Part model, mm, in its own coordinate system. Face numbers are marked on the shaded views. A direction names the side the tool comes from. Give positions to 0.01 mm unless a question says otherwise; leave off trailing zeros. Order: outer loops, then holes, each group sorted by start corner. A loop starts at its lowest first (then second) coordinate and runs counter-clockwise, first axis right, second up. Notation, with made-up numbers: (51, 2.25) - (84, 2.25) arc R7 ccw to (84, 11.25) - close; hole circle Ø2 at (77.5, 5). An arc over 180 degrees is marked (long way). Use a Markdown table: item, result. Add a question column.
from build123d import *

# Parameters (mm, degrees)
F1_W     = 83
F1_H     = 83
F1_W_2   = 73
F1_H_2   = 73
F2_DEPTH = 2
F3_W     = 75
F3_H     = 75
F4_DEPTH = 5


# Not quite as in the source:
# - a feature names something its author has since deleted; it is built from what else it names


with BuildPart() as f2:
    # F1 (on Front) → F2 (new body)
    with BuildSketch(Plane.XZ):
        with Locations((-0.3727272727, 0)):
            Rectangle(F1_W, F1_H)
        with Locations((-0.3727272727, 0)):
            Rectangle(F1_W_2, F1_H_2, mode=Mode.SUBTRACT)
    extrude(amount=F2_DEPTH)

    # F3 (on face) → F4 (join)
    with BuildSketch(Plane.XZ.offset(2)):
        with Locations((-0.3727272727, 0)):
            Rectangle(F3_W, F3_H)
    extrude(amount=F4_DEPTH)


solid = f2.part
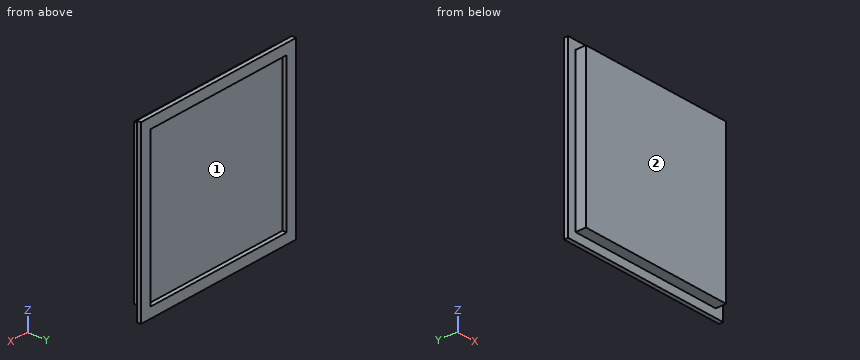
1. Pin check, flat tips, straight feed: P1, Ø1.5, axis at y = -5, z = 30.5, coming from the -X side; P2, Ø4, axis at x = -8.5, y = -5.5, coming from the -Z side; P3, Ø4, axis at x = -29, y = -6.5, coming from the +Z side; P4, Ø3, axis at y = -2.5, z = 15, coming from the -X side. Stop position of each tip, or through.
2. Cut at B-B (x = -35.5). Write the cut outline in (y, z), plus the area to 3 significant figures.
3. Drill centre lines: probe 1 along Z at (x, y) = (17.5, -0.25); probe 2 along X at (y, z) = (-0.75, -17.5); probe 3 along Z at (x, y) = (-16, -5.5). Where is each one in solid material? Low to high. Write a range as [from, to].
4. Tool access for the marked faces 1 and 2: list every direction of +Z, -Z, +X, -X, +Y, -Y with a clear straight run to the whole face (end or side of a thin tool).
5. Cut at A-A (z = -20.5). Write the cut outline in (x, y), plus the area to 3 significant figures.
6. Cut at C-C (y = -4). Write the cut outline in (x, z).
Responses:
| question | item | result |
|---|---|---|
| 1 | P1 | stops at x = -37.87 |
| 1 | P2 | stops at z = -37.5 |
| 1 | P3 | stops at z = 37.5 |
| 1 | P4 | stops at x = -41.87 |
| 2 | outline | (-7, -37.5) - (-2, -37.5) - (-2, -41.5) - (0, -41.5) - (0, -36.5) - (-2, -36.5) - (-2, 36.5) - (0, 36.5) - (0, 41.5) - (-2, 41.5) - (-2, 37.5) - (-7, 37.5) - close |
| 2 | area | 395 mm² |
| 3 | probe 1 | z = [-41.5, -36.5], [36.5, 41.5] |
| 3 | probe 2 | x = [-41.87, -36.87], [36.13, 41.13] |
| 3 | probe 3 | z = [-37.5, 37.5] |
| 4 | face 1 | +Y |
| 4 | face 2 | +Z, -Z, +X, -X, -Y |
| 5 | outline | (-41.87, -2) - (-37.87, -2) - (-37.87, -7) - (37.13, -7) - (37.13, -2) - (41.13, -2) - (41.13, 0) - (36.13, 0) - (36.13, -2) - (-36.87, -2) - (-36.87, 0) - (-41.87, 0) - close |
| 5 | area | 395 mm² |
| 6 | outline | (-37.87, -37.5) - (37.13, -37.5) - (37.13, 37.5) - (-37.87, 37.5) - close |
